Source: CAD feature listing. Evaluate the final solid. Frame: model axes, mm. Give positions to 0.01 mm unless a question says otherwise; leave off trailing zeros. Write each loop counter-clockwise with the first axis right and the second up, starting at its lowest first coordinate (ties: lowest second). Pieces come first, ordered by that corner, then holes. Notation, with made-up numbers: (68, 27) -> (123, 27) arc R8 ccw to (123, 32) -> close; hole circle Ø5 at (81, -4.75). An arc over 180 degrees is marked (long way). Use one line per item in the form item = value. Start each with the question number.
(1) Cut plane C-C, the plane z = -88.9. Output: boundary loops of the cut face in (x, y) (3 decimals).
(2) Draft query along Y for faces 1 (the face through (52, -2, -25.4)), 2 (the face through (50, 0, -57)), 3 (the face through (50, -3.175, -57)). Return one class per face: pulls with the +Y half, pulls with the -Y half, needs draft (parallel to the pull), parting line crosses it, or undercut.
(3) Material intervals for line 1 along Z through (x, y) = (50.8, -1.65); line 2 along X through (y, z) = (-1.95, -84.5); line 3 along X through (y, z) = (-3, -85.5), sorted ascending. Write a range as from..to.
(4) Cut plane B-B, the plane y = -1.7. Output: boundary loops of the cut face in (x, z), and give its area (3 significant figures).
(5) Cut plane D-D, the plane x = 86. Output: boundary loops of the cut face in (y, z) (3 decimals).
(6) First-contact query: P1, Ø10, axis at x = 50.8, z = -88.9, coming from the -Y side. Flat tip, straight axial feed; report the tip coordinate or a pass-through.
(7) Cut plane A-A, the plane x = 50.8. Output: boundary loops of the cut face in (y, z) (3 decimals).
from build123d import *

# Parameters (mm, degrees)
F0_R     = 6.35
F1_DEPTH = 3.175


with BuildPart() as f1:
    # F0 (on Front) → F1 (new body)
    with BuildSketch(Plane.XZ):
        Polygon((101.6, -25.4), (0, -25.4), (0, -69.85), (50.8, -69.85), (101.6, -69.85), align=None)
        with BuildLine():
            Line((50.8, -69.85), (0, -69.85))
            Line((0, -69.85), (38.273973, -103.25274))
            ThreePointArc((38.273973, -103.25274), (32.962929, -82.211098), (50.8, -69.85))
        make_face()
        with BuildLine():
            Line((63.326027, -103.25274), (101.6, -69.85))
            Line((101.6, -69.85), (50.8, -69.85))
            ThreePointArc((50.8, -69.85), (64.270384, -75.429616), (69.85, -88.9))
            ThreePointArc((69.85, -88.9), (68.142481, -96.782946), (63.326027, -103.25274))
        make_face()
        with BuildLine():
            ThreePointArc((69.85, -88.9), (64.270384, -75.429616), (50.8, -69.85))
            ThreePointArc((50.8, -69.85), (32.962929, -82.211098), (38.273973, -103.25274))
            ThreePointArc((38.273973, -103.25274), (50.8, -107.95), (63.326027, -103.25274))
            ThreePointArc((63.326027, -103.25274), (68.142481, -96.782946), (69.85, -88.9))
        make_face()
        with Locations((50.8, -88.9)):
            Circle(F0_R, mode=Mode.SUBTRACT)
    extrude(amount=F1_DEPTH)


solid = f1.part
Geometry says:
q1.outline = (21.828, -3.175) -> (44.45, -3.175) -> (44.45, 0) -> (21.828, 0) -> close; (57.15, -3.175) -> (79.772, -3.175) -> (79.772, 0) -> (57.15, 0) -> close
q2.face_1 = needs draft
q2.face_2 = pulls with the +Y half
q2.face_3 = pulls with the -Y half
q3.line_1 = -107.95..-95.25, -82.55..-25.4
q3.line_2 = 16.79..46.22, 55.38..84.81
q3.line_3 = 17.93..45.44, 56.16..83.67
q4.outline = (0, -69.85) -> (38.27, -103.25) arc R19.05 ccw to (63.33, -103.25) -> (101.6, -69.85) -> (101.6, -25.4) -> (0, -25.4) -> close; hole circle Ø12.7 at (50.8, -88.9)
q4.area = 6,590 mm^2
q5.outline = (-3.175, -83.465) -> (0, -83.465) -> (0, -25.4) -> (-3.175, -25.4) -> close
q6.P1 = through
q7.outline = (-3.175, -107.95) -> (0, -107.95) -> (0, -95.25) -> (-3.175, -95.25) -> close; (-3.175, -82.55) -> (0, -82.55) -> (0, -25.4) -> (-3.175, -25.4) -> close
